Could you check a few things on this model? Use its own coordinates, in mm. A direction names the side the tool comes from. Give positions to 0.01 mm unless a question says otherwise; leave off trailing zeros. Loops run counter-clockwise (first coordinate to the right, second up) from the corner with the lowest first, then second, coordinate; pieces in that order, holes last. Notation, with made-up numbers: M 80,62 L 121,62 A11 cw 121,69 Z; hole C -20.75,66.5 d8. An arc over 180 degrees is marked long. Return JSON: item names as keys, results as strings. Group by question number.
1. Please list where these lines run through material, in increasing order: line 1 (Y direction, x = 32.5, z = 0.7); line 2 (Y direction, x = -58.5, z = 0.95); line 3 (Y direction, x = -77.5, z = 1.2).
2. For pin 1 (1.5 mm diameter, centred on y = 2, z = 1.5, fed in from -X); pin 2 (0.9 mm diameter, centred on x = -46.5, z = 2, fed in from -Y), each with a flat end and sliding along its axis, tell me the tip position at first contact or that it passes through.
3. If we section it at C-C (z = 0.8): State how many separate pieces and enclosed holes the cut face has, plus the area to 3 significant figures.
4. If we section it at A-A (x = -15): Write out the boundary of the cut face in (y, z), plus the area to 3 significant figures.
5. If we mould it in two halves opening along X, with no side actions, what happens to faces 1 (the cylindrical face through (87.15, -11.99, 1.52)), 2 (the cylindrical face through (-56.653, -0.766, 1.521)), 3 (the cylindrical face through (84.408, 5.601, 1.521)), 4 (the flat face through (-1, 0, 3))? For each: +X half, -X half, draft (parallel to the pull), parting line (faces both ways), or undercut.
6. For faces 5 (the flat face through (57, -10.25, 2)), 6 (the flat face through (90, 0, 1)), 7 (the flat face through (27, 13, 1)), 8 (the flat face through (-24, -11, 1)), 9 (the cylindrical face through (87.15, 11.99, 1.52)), which set-ups out of +Z, -Z, +X, -X, +Y, -Y let a thin tool reach every point of the face, with its end or its side?
7. If we section it at D-D (x = 32.5): Write out the boundary of the cut face in (y, z).
8. If we section it at B-B (y = 0): Write out the boundary of the cut face in (x, z), plus the area to 4 significant figures.
```python
from build123d import *

# Parameters (mm, degrees)
SALIENTE_EXTRUIR1_DEPTH = 3
REDONDEO1_R             = 10
CHAFL_N1_SIZE           = 4
CORTAR_EXTRUIR1_REACH   = 93.291
CROQUIS2_R              = 2
CROQUIS2_W              = 40.5
CROQUIS2_H              = 20.5
CORTAR_EXTRUIR2_REACH   = 93.291
CROQUIS3_R              = 3.5
CROQUIS3_R_2            = 2
CORTAR_EXTRUIR3_REACH   = 93.291
CROQUIS4_R              = 2


with BuildPart() as part:
    # Croquis1 → Saliente-Extruir1 (new body)
    with BuildSketch(Plane.XY):
        with BuildLine():
            Line((90, -15), (90, 15))
            Line((90, 15), (25, 15))
            Line((25, 15), (25, 11))
            Line((25, 11), (-25, 11))
            Line((-25, 11), (-71.562828956, 11))
            ThreePointArc((-71.562828956, 11), (-90, 0), (-71.562828956, -11))
            Line((-71.562828956, -11), (-25, -11))
            Line((-25, -11), (25, -11))
            Line((25, -11), (25, -15))
            Line((25, -15), (90, -15))
        make_face()
    extrude(amount=SALIENTE_EXTRUIR1_DEPTH)

    # Redondeo1
    redondeo1_edges = [part.edges().sort_by_distance(p)[0] for p in [
        (90, 15, 1.5),
        (90, -15, 1.5),
    ]]
    fillet(redondeo1_edges, radius=REDONDEO1_R)

    # Chaflán1
    chafl_n1_edges = [part.edges().sort_by_distance(p)[0] for p in [
        (25, -15, 1.5),
        (25, 15, 1.5),
    ]]
    chamfer(chafl_n1_edges, length=CHAFL_N1_SIZE - 0.0001)  # a hair under: the kernel refuses the full size

    # Croquis2 → Cortar-Extruir1 (cut, up to next)
    with BuildSketch(Plane.XY.offset(3), mode=Mode.PRIVATE) as cortar_extruir1_sk1:
        with Locations((82.5, 5)):
            Circle(CROQUIS2_R)
    cortar_extruir1_tool1 = extrude(cortar_extruir1_sk1.sketch, amount=-CORTAR_EXTRUIR1_REACH, mode=Mode.PRIVATE) & part.part
    # Croquis2 → Cortar-Extruir1 (cut, up to next)
    with BuildSketch(Plane.XY.offset(3), mode=Mode.PRIVATE) as cortar_extruir1_sk2:
        with Locations((32.5, 5)):
            Circle(CROQUIS2_R)
    cortar_extruir1_tool2 = extrude(cortar_extruir1_sk2.sketch, amount=-CORTAR_EXTRUIR1_REACH, mode=Mode.PRIVATE) & part.part
    # Croquis2 → Cortar-Extruir1 (cut, up to next)
    with BuildSketch(Plane.XY.offset(3), mode=Mode.PRIVATE) as cortar_extruir1_sk3:
        with Locations((82.5, -5)):
            Circle(CROQUIS2_R)
    cortar_extruir1_tool3 = extrude(cortar_extruir1_sk3.sketch, amount=-CORTAR_EXTRUIR1_REACH, mode=Mode.PRIVATE) & part.part
    # Croquis2 → Cortar-Extruir1 (cut, up to next)
    with BuildSketch(Plane.XY.offset(3), mode=Mode.PRIVATE) as cortar_extruir1_sk4:
        with Locations((32.5, -5)):
            Circle(CROQUIS2_R)
    cortar_extruir1_tool4 = extrude(cortar_extruir1_sk4.sketch, amount=-CORTAR_EXTRUIR1_REACH, mode=Mode.PRIVATE) & part.part
    # Croquis2 → Cortar-Extruir1 (cut, up to next)
    with BuildSketch(Plane.XY.offset(3), mode=Mode.PRIVATE) as cortar_extruir1_sk5:
        with Locations((57.5, 0)):
            Rectangle(CROQUIS2_W, CROQUIS2_H)
    cortar_extruir1_tool5 = extrude(cortar_extruir1_sk5.sketch, amount=-CORTAR_EXTRUIR1_REACH, mode=Mode.PRIVATE) & part.part
    add(cortar_extruir1_tool1.solids().sort_by_distance((82.5, 5, 3))[0], mode=Mode.SUBTRACT)
    add(cortar_extruir1_tool2.solids().sort_by_distance((32.5, 5, 3))[0], mode=Mode.SUBTRACT)
    add(cortar_extruir1_tool3.solids().sort_by_distance((82.5, -5, 3))[0], mode=Mode.SUBTRACT)
    add(cortar_extruir1_tool4.solids().sort_by_distance((32.5, -5, 3))[0], mode=Mode.SUBTRACT)
    add(cortar_extruir1_tool5.solids().sort_by_distance((57.5, 0, 3))[0], mode=Mode.SUBTRACT)

    # Croquis3 → Cortar-Extruir2 (cut, up to next)
    with BuildSketch(Plane.XY.offset(3), mode=Mode.PRIVATE) as cortar_extruir2_sk1:
        with Locations((-77.5, 0)):
            Circle(CROQUIS3_R)
    cortar_extruir2_tool1 = extrude(cortar_extruir2_sk1.sketch, amount=-CORTAR_EXTRUIR2_REACH, mode=Mode.PRIVATE) & part.part
    # Croquis3 → Cortar-Extruir2 (cut, up to next)
    with BuildSketch(Plane.XY.offset(3), mode=Mode.PRIVATE) as cortar_extruir2_sk2:
        with Locations((-58.5, 0)):
            Circle(CROQUIS3_R_2)
    cortar_extruir2_tool2 = extrude(cortar_extruir2_sk2.sketch, amount=-CORTAR_EXTRUIR2_REACH, mode=Mode.PRIVATE) & part.part
    add(cortar_extruir2_tool1.solids().sort_by_distance((-77.5, 0, 3))[0], mode=Mode.SUBTRACT)
    add(cortar_extruir2_tool2.solids().sort_by_distance((-58.5, 0, 3))[0], mode=Mode.SUBTRACT)

    # Croquis4 → Cortar-Extruir3 (cut, up to next)
    with BuildSketch(Plane.XY.offset(3), mode=Mode.PRIVATE) as cortar_extruir3_sk1:
        with Locations((-15, 0)):
            Circle(CROQUIS4_R)
    cortar_extruir3_tool1 = extrude(cortar_extruir3_sk1.sketch, amount=-CORTAR_EXTRUIR3_REACH, mode=Mode.PRIVATE) & part.part
    # Croquis4 → Cortar-Extruir3 (cut, up to next)
    with BuildSketch(Plane.XY.offset(3), mode=Mode.PRIVATE) as cortar_extruir3_sk2:
        with Locations((15, 0)):
            Circle(CROQUIS4_R)
    cortar_extruir3_tool2 = extrude(cortar_extruir3_sk2.sketch, amount=-CORTAR_EXTRUIR3_REACH, mode=Mode.PRIVATE) & part.part
    add(cortar_extruir3_tool1.solids().sort_by_distance((-15, 0, 3))[0], mode=Mode.SUBTRACT)
    add(cortar_extruir3_tool2.solids().sort_by_distance((15, 0, 3))[0], mode=Mode.SUBTRACT)


solid = part.part
```
Answer:
{
 "1": {"line 1": "y = -15 to -7, -3 to 3, 7 to 15", "line 2": "y = -11 to -2, 2 to 11", "line 3": "y = -12.5 to -3.5, 3.5 to 12.5"},
 "2": {"pin 1": "stops at x = -89.94", "pin 2": "stops at y = -11"},
 "3": {"separate pieces": "1", "enclosed holes": "9", "area": "3,450 mm²"},
 "4": {"outline": "M -11,0 L -2,0 L -2,3 L -11,3 Z; M 2,0 L 11,0 L 11,3 L 2,3 Z", "area": "54.0 mm²"},
 "5": {"face 1": "+X half", "face 2": "undercut", "face 3": "undercut", "face 4": "draft"},
 "6": {"face 5": "+Z, -Z", "face 6": "+Z, -Z, +X, +Y, -Y", "face 7": "+Z, -Z, +Y", "face 8": "+Z, -Z, -Y", "face 9": "+Z, -Z, +X, +Y"},
 "7": {"outline": "M -15,0 L -7,0 L -7,3 L -15,3 Z; M -3,0 L 3,0 L 3,3 L -3,3 Z; M 7,0 L 15,0 L 15,3 L 7,3 Z"},
 "8": {"outline": "M -90,0 L -81,0 L -81,3 L -90,3 Z; M -74,0 L -60.5,0 L -60.5,3 L -74,3 Z; M -56.5,0 L -17,0 L -17,3 L -56.5,3 Z; M -13,0 L 13,0 L 13,3 L -13,3 Z; M 17,0 L 37.25,0 L 37.25,3 L 17,3 Z; M 77.75,0 L 90,0 L 90,3 L 77.75,3 Z", "area": "361.5 mm²"}
}
